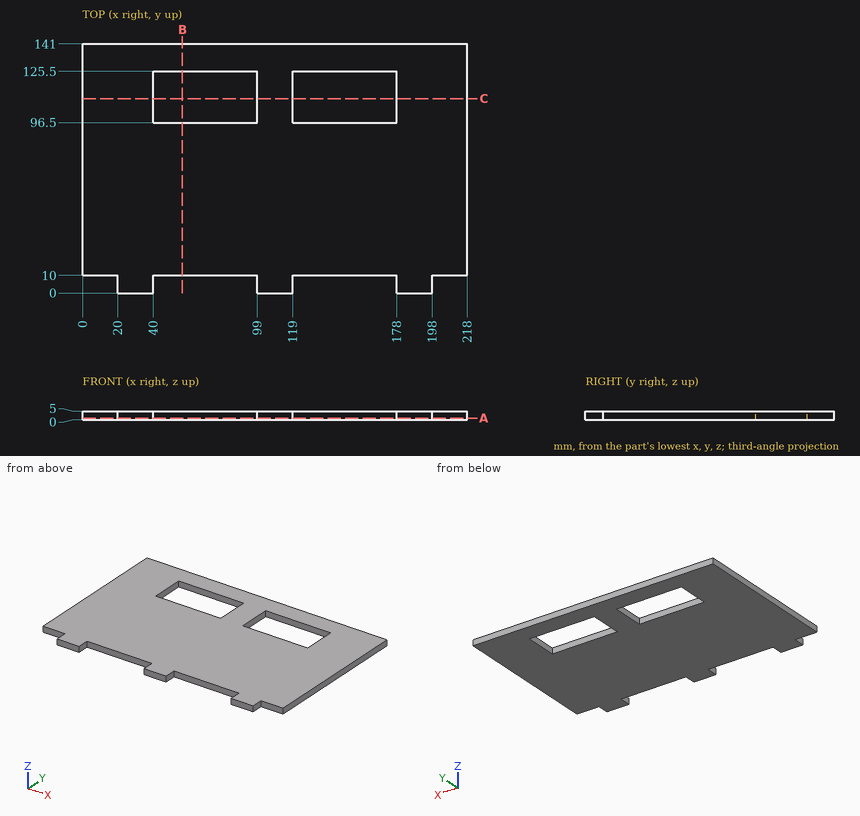
Print and shaded views of the part. All mm, measured from the part's lowest x, y and z. Give positions to 0.01 mm unless a question says otherwise; leave off trailing zeros. Write each loop counter-clockwise with the first axis right and the second up, starting at its lowest first coordinate (ties: lowest second). Pieces come first, ordered by that corner, then holes. Notation, with made-up numbers: (-18, 46) -> (13, 46) arc R9 ccw to (13, 58) -> close; hole circle Ø1 at (74.25, -27.5). An arc over 180 degrees is marked (long way). Write each question's results on one line, items separated by ' | '.
1. Drop flat-ended pins along their axis: P1, Ø1.5, axis at x = 158.5, z = 2, coming from the -Y side; P2, Ø2.5, axis at y = 3.5, z = 3, coming from the -X side; P3, Ø2.5, axis at y = 6.5, z = 2, coming from the +X side. Give the stop position or say it passes through.
Geometry check:
P1: y = 10 | P2: x = 20 | P3: x = 198
2. Cut at B-B, the plane x = 56.5. Write the cut outline in (y, z), then the cut area to 3 significant figures.
Geometry check:
outline: (10, 0) -> (96.5, 0) -> (96.5, 5) -> (10, 5) -> close; (125.5, 0) -> (141, 0) -> (141, 5) -> (125.5, 5) -> close | area: 510 mm²
3. Cut at A-A, the plane z = 0.9. Write the cut outline in (x, y).
Geometry check:
outline: (0, 10) -> (20, 10) -> (20, 0) -> (40, 0) -> (40, 10) -> (99, 10) -> (99, 0) -> (119, 0) -> (119, 10) -> (178, 10) -> (178, 0) -> (198, 0) -> (198, 10) -> (218, 10) -> (218, 141) -> (0, 141) -> close; hole (40, 96.5) -> (99, 96.5) -> (99, 125.5) -> (40, 125.5) -> close; hole (119, 96.5) -> (178, 96.5) -> (178, 125.5) -> (119, 125.5) -> close
4. Wall check: probe 1 along X at (y, z) = (8, 1.15); probe 2 along X at (y, z) = (114, 3.9); probe 3 along Y at (x, z) = (159.5, 2.65). Give the ranges that are in metal, low to high. Write a range as [from, to].
Geometry check:
probe 1: [20, 40], [99, 119], [178, 198] | probe 2: [0, 40], [99, 119], [178, 218] | probe 3: [10, 96.5], [125.5, 141]
5. Cut at C-C, the plane y = 110. Write the cut outline in (x, z), then the cut area to 3 significant figures.
Geometry check:
outline: (0, 0) -> (40, 0) -> (40, 5) -> (0, 5) -> close; (99, 0) -> (119, 0) -> (119, 5) -> (99, 5) -> close; (178, 0) -> (218, 0) -> (218, 5) -> (178, 5) -> close | area: 500 mm²
